```python
from build123d import *

# Parameters (mm, degrees)
SKETCH1_W           = 20
SKETCH1_H           = 20
BOSS_EXTRUDE1_DEPTH = 20
SKETCH2_R           = 5.520822916
BOSS_EXTRUDE3_DEPTH = 30
BOSS_EXTRUDE4_DEPTH = 0.1
SKETCH4_W           = 2.557692308
SKETCH4_H           = 0.314102564
BOSS_EXTRUDE5_DEPTH = 0.1


with BuildPart() as part:
    # Sketch1 → Boss-Extrude1 (new body)
    with BuildSketch(Plane.XY):
        with Locations((-10, 10)):
            Rectangle(SKETCH1_W, SKETCH1_H)
    extrude(amount=BOSS_EXTRUDE1_DEPTH)

    # Sketch2 → Boss-Extrude3 (add)
    with BuildSketch(Plane(origin=(0, 0, 0), x_dir=(1, 0, 0), z_dir=(0, 1, 0))):
        with Locations((-10, -10)):
            Circle(SKETCH2_R)
    extrude(amount=BOSS_EXTRUDE3_DEPTH)

    # Sketch3 → Boss-Extrude4 (add)
    with BuildSketch(Plane(origin=(0, 30, 0), x_dir=(1, 0, 0), z_dir=(0, 1, 0))):
        with BuildLine():
            Line((-8.325722208, -8.914299791), (-8.588642881, -9.077661169))
            add(Edge.make_bspline(
                [(-8.588642881, -9.077661169), (-8.617472747, -9.041832775), (-8.674219442, -8.971310665), (-8.772758678, -8.880300732), (-8.877770093, -8.80213369), (-8.99104814, -8.738429939), (-9.11243394, -8.689208489), (-9.241448792, -8.654378283), (-9.378074297, -8.63267404), (-9.471739496, -8.630207204), (-9.519732625, -8.628943221)],
                knots=[0, 0, 0, 0, 1.026593902, 2.0206758, 2.988051866, 3.946915611, 4.916868779, 5.907761954, 6.927957743, 8, 8, 8, 8], degree=3))
            add(Edge.make_bspline(
                [(-9.519732625, -8.628943221), (-9.558091582, -8.630000063), (-9.633638505, -8.632081485), (-9.744544658, -8.645091978), (-9.850187011, -8.668733986), (-9.95122772, -8.699884943), (-10.046948139, -8.741635233), (-10.137599057, -8.792444989), (-10.223984547, -8.85149503), (-10.303601288, -8.919905575), (-10.376430295, -8.994304243), (-10.439529209, -9.074057938), (-10.494466143, -9.156777829), (-10.537572099, -9.244529571), (-10.572847269, -9.335305625), (-10.59605399, -9.43081948), (-10.611518685, -9.529847488), (-10.613288014, -9.597365828), (-10.614183747, -9.631547387)],
                knots=[0, 0, 0, 0, 1.112346261, 2.190735716, 3.231507886, 4.247384806, 5.251966152, 6.253067467, 7.256802811, 8.280671706, 9.291813951, 10.270744147, 11.225547591, 12.165006084, 13.100104208, 14.043489273, 15.009504848, 16, 16, 16, 16], degree=3))
            add(Edge.make_bspline(
                [(-10.614183747, -9.631547387), (-10.612404495, -9.676316598), (-10.608869964, -9.765251794), (-10.581168504, -9.896529896), (-10.535824097, -10.023453586), (-10.473766246, -10.145121723), (-10.395289112, -10.257715879), (-10.303116549, -10.358699333), (-10.197197465, -10.446115361), (-10.078465135, -10.518587886), (-9.949707391, -10.576849254), (-9.812317286, -10.618356587), (-9.667417506, -10.643408959), (-9.568210759, -10.646564902), (-9.51762926, -10.64817399)],
                knots=[0, 0, 0, 0, 0.966302908, 1.919585723, 2.883856336, 3.870342332, 4.860282998, 5.839159637, 6.814385684, 7.815993281, 8.834850808, 9.858348828, 10.908058873, 12, 12, 12, 12], degree=3))
            add(Edge.make_bspline(
                [(-9.51762926, -10.64817399), (-9.471274075, -10.646874493), (-9.380173837, -10.644320636), (-9.247006552, -10.622791672), (-9.120226641, -10.587548039), (-8.99983861, -10.538400389), (-8.886062444, -10.474872873), (-8.779633269, -10.396513702), (-8.678433331, -10.305577102), (-8.618936355, -10.23525913), (-8.588642881, -10.199456041)],
                knots=[0, 0, 0, 0, 1.039848629, 2.043578496, 3.018386758, 3.987534228, 4.954977003, 5.934852016, 6.948509513, 8, 8, 8, 8], degree=3))
            Line((-8.588642881, -10.199456041), (-8.325722208, -10.371932003))
            add(Edge.make_bspline(
                [(-8.325722208, -10.371932003), (-8.341309911, -10.39482273), (-8.372433577, -10.440528206), (-8.424461203, -10.504972323), (-8.480581035, -10.565294005), (-8.540574131, -10.621412395), (-8.603657141, -10.674670415), (-8.671985051, -10.722521989), (-8.743354662, -10.767656812), (-8.81860382, -10.808269684), (-8.896954518, -10.844776005), (-8.978296508, -10.876167176), (-9.06227632, -10.903137282), (-9.148992697, -10.924574629), (-9.238616595, -10.941685467), (-9.330916229, -10.953039169), (-9.425859811, -10.96151445), (-9.490031962, -10.962020317), (-9.522537112, -10.962276554)],
                knots=[0, 0, 0, 0, 0.954134338, 1.905101784, 2.851144739, 3.791306361, 4.734911809, 5.6936923, 6.663572882, 7.643865596, 8.638447847, 9.640600242, 10.646758161, 11.676244097, 12.717260333, 13.78922464, 14.880174919, 16, 16, 16, 16], degree=3))
            add(Edge.make_bspline(
                [(-9.522537112, -10.962276554), (-9.572147996, -10.961385274), (-9.669385688, -10.959638359), (-9.811708196, -10.940429884), (-9.947721863, -10.911472268), (-10.077380221, -10.869908534), (-10.200703455, -10.816403758), (-10.317576573, -10.751046844), (-10.427612591, -10.673295054), (-10.529723374, -10.584532285), (-10.62350482, -10.488291644), (-10.704031011, -10.384441726), (-10.773876281, -10.276800678), (-10.829963824, -10.162991152), (-10.874610751, -10.044525779), (-10.905115583, -9.920455539), (-10.924845321, -9.791803285), (-10.927128701, -9.704070403), (-10.928286311, -9.659592259)],
                knots=[0, 0, 0, 0, 1.1129367, 2.181364009, 3.217532258, 4.231199276, 5.232079859, 6.230262199, 7.231623845, 8.250719726, 9.263571943, 10.242672461, 11.195837495, 12.138959767, 13.085126421, 14.0317438, 15.002148558, 16, 16, 16, 16], degree=3))
            add(Edge.make_bspline(
                [(-10.928286311, -9.659592259), (-10.927845295, -9.629413825), (-10.926968041, -9.569383937), (-10.916906113, -9.48028887), (-10.90390764, -9.392380325), (-10.881881903, -9.306772606), (-10.856441271, -9.222167316), (-10.82396574, -9.139584214), (-10.785870345, -9.058639542), (-10.742618397, -8.979541812), (-10.693929652, -8.903592273), (-10.640048419, -8.831838608), (-10.583004083, -8.763418842), (-10.520127971, -8.700695082), (-10.454088317, -8.64115889), (-10.383016741, -8.586400766), (-10.30732089, -8.536259775), (-10.228137567, -8.48980876), (-10.145512856, -8.448449325), (-10.059946185, -8.412816087), (-9.971953156, -8.382363511), (-9.881393012, -8.358254592), (-9.788866839, -8.338037168), (-9.693645501, -8.325319322), (-9.596093279, -8.316333049), (-9.530037256, -8.315342257), (-9.496595606, -8.314840657)],
                knots=[0, 0, 0, 0, 0.990994727, 1.971252077, 2.943264845, 3.907940874, 4.872158414, 5.844625996, 6.82015047, 7.809835459, 8.804511986, 9.781214284, 10.756496977, 11.728388426, 12.696359165, 13.676225489, 14.672885716, 15.677705647, 16.690706858, 17.706033469, 18.721040654, 19.747369689, 20.783475414, 21.830280724, 22.901553713, 24, 24, 24, 24], degree=3))
            add(Edge.make_bspline(
                [(-9.496595606, -8.314840657), (-9.454715498, -8.315762548), (-9.371164618, -8.317601722), (-9.247223911, -8.333080374), (-9.125108718, -8.35641679), (-9.006961614, -8.39098962), (-8.8942151, -8.432853276), (-8.788679649, -8.47986599), (-8.692839546, -8.534460594), (-8.604911956, -8.594180708), (-8.524732439, -8.661541614), (-8.451477947, -8.737348571), (-8.383646297, -8.82120705), (-8.345189586, -8.883012781), (-8.325722208, -8.914299791)],
                knots=[0, 0, 0, 0, 1.095225653, 2.184976855, 3.262915854, 4.344593502, 5.400796181, 6.407717688, 7.363229445, 8.282371371, 9.184954523, 10.097238608, 11.036792983, 12, 12, 12, 12], degree=3))
        make_face()
    extrude(amount=BOSS_EXTRUDE4_DEPTH)

    # Sketch4 → Boss-Extrude5 (add)
    with BuildSketch(Plane(origin=(0, 30, 0), x_dir=(1, 0, 0), z_dir=(0, 1, 0))):
        with BuildLine():
            add(Edge.make_bspline(
                [(-6.365384615, -9.892828526), (-6.36629269, -9.912316587), (-6.368070874, -9.950477954), (-6.383176643, -10.005717448), (-6.409172417, -10.055966244), (-6.442915564, -10.101200835), (-6.484230683, -10.138698232), (-6.53117379, -10.165585861), (-6.58227867, -10.182750842), (-6.617887461, -10.184835854), (-6.636017628, -10.185897436)],
                knots=[0, 0, 0, 0, 1.054986045, 2.065865298, 3.074122704, 4.105114675, 5.109626121, 6.074217918, 7.019490725, 8, 8, 8, 8], degree=3))
            add(Edge.make_bspline(
                [(-6.636017628, -10.185897436), (-6.653677192, -10.184812106), (-6.688588061, -10.182666538), (-6.738806847, -10.16559855), (-6.785096281, -10.138472811), (-6.826330626, -10.101225793), (-6.86005428, -10.055959652), (-6.886055203, -10.005719191), (-6.901159612, -9.950477495), (-6.902937984, -9.912316432), (-6.903846154, -9.892828526)],
                knots=[0, 0, 0, 0, 0.961106377, 1.899993565, 2.859409042, 3.870007927, 4.90724781, 5.921615355, 6.938620636, 8, 8, 8, 8], degree=3))
            add(Edge.make_bspline(
                [(-6.903846154, -9.892828526), (-6.902967151, -9.873564442), (-6.901256287, -9.836069421), (-6.885874492, -9.78184562), (-6.860110821, -9.732405344), (-6.825863936, -9.687910508), (-6.785370463, -9.649925015), (-6.738771881, -9.622899362), (-6.688596963, -9.60578574), (-6.653680183, -9.603646321), (-6.636017628, -9.602564103)],
                knots=[0, 0, 0, 0, 1.055304112, 2.054011575, 3.063363921, 4.096942562, 5.122536081, 6.088009498, 7.032825006, 8, 8, 8, 8], degree=3))
            add(Edge.make_bspline(
                [(-6.636017628, -9.602564103), (-6.617884357, -9.603622457), (-6.582269469, -9.605701133), (-6.531209353, -9.622912645), (-6.483954162, -9.649696813), (-6.443381916, -9.687935052), (-6.409116, -9.732398919), (-6.383357305, -9.781847293), (-6.36797421, -9.836068977), (-6.366263526, -9.873564292), (-6.365384615, -9.892828526)],
                knots=[0, 0, 0, 0, 0.986662878, 1.937868148, 2.908513651, 3.927890639, 4.955204348, 5.958438607, 6.951092507, 8, 8, 8, 8], degree=3))
        make_face()
        with Locations((-8.721153846, -9.894230769)):
            Rectangle(SKETCH4_W, SKETCH4_H)
    extrude(amount=BOSS_EXTRUDE5_DEPTH)


solid = part.part
```
Work out the finished part from the listing and answer in its coordinate system (mm). A direction names the side the tool comes from. Coordinates: 2 decimals unless noted, no trailing zeros. Loops run counter-clockwise (first coordinate to the right, second up) from the corner with the lowest first, then second, coordinate; pieces in that order, holes last. Notation, with made-up numbers: (63.5, 25) - (102.5, 25) arc R29 cw to (102.5, 53) - close; hole circle Ø4 at (15, 52.25). An arc over 180 degrees is marked (long way). Use a Markdown table: item, result.
Item 1: For faces 1 (the cylindrical face through (-7.452, 24.93, 14.898)), 2 (the flat face through (-10, 10, 20)), determine the directions among +Z, -Z, +X, -X, +Y, -Y from which every point of the face is accessible in a straight line to the end or side of a thin tool.
Evaluation:
| item | result |
|---|---|
| face 1 | +Y |
| face 2 | +Z, +X, -X, +Y, -Y |
Item 2: Find section B-B, the plane x = -12.5. Determine the outline of the cut face in (y, z), and give its area (3 significant figures).
Evaluation:
| item | result |
|---|---|
| outline | (0, 0) - (20, 0) - (20, 5.08) - (30, 5.08) - (30, 14.92) - (20, 14.92) - (20, 20) - (0, 20) - close |
| area | 498 mm2 |
Item 3: Consider probe 1 along Y at (x, z) = (-16.25, 14.5); probe 2 along Z at (x, y) = (-12, 22); probe 3 along Z at (x, y) = (-14, 28). Determine where each line is inside the solid, lowest interval first. Write a range as from..to.
Evaluation:
| item | result |
|---|---|
| probe 1 | y = 0..20 |
| probe 2 | z = 4.85..15.15 |
| probe 3 | z = 6.19..13.81 |
Item 4: Find section A-A, the plane z = 12. Determine the outline of the cut face in (x, y), and give its area (3 significant figures).
Evaluation:
| item | result |
|---|---|
| outline | (-20, 0) - (0, 0) - (0, 20) - (-4.85, 20) - (-4.85, 30) - (-15.15, 30) - (-15.15, 20) - (-20, 20) - close |
| area | 503 mm2 |
Item 5: Find section C-C, the plane y = 21.5. Determine the outline of the cut face in (x, z).
Evaluation:
| item | result |
|---|---|
| outline | circle Ø11.04 at (-10, 10) |
Item 6: Find section D-D, the plane z = 17.75. Determine the outline of the cut face in (x, y), and give its area (3 significant figures).
Evaluation:
| item | result |
|---|---|
| outline | (-20, 0) - (0, 0) - (0, 20) - (-20, 20) - close |
| area | 400 mm2 |
Item 7: Given pin 1 Ø4 at (x, z) = (-3.5, 12.5) entering from +Y; pin 2 Ø5.5 at (x, z) = (-12.5, 11) entering from +Y; pin 3 Ø3 at (x, z) = (-7, 17.5) entering from +Y, each flat-ended and moving along its own axis, determine where each tip first touches the part or whether it passes through.
Evaluation:
| item | result |
|---|---|
| pin 1 | stops at y = 30 |
| pin 2 | stops at y = 30.1 |
| pin 3 | stops at y = 20 |
